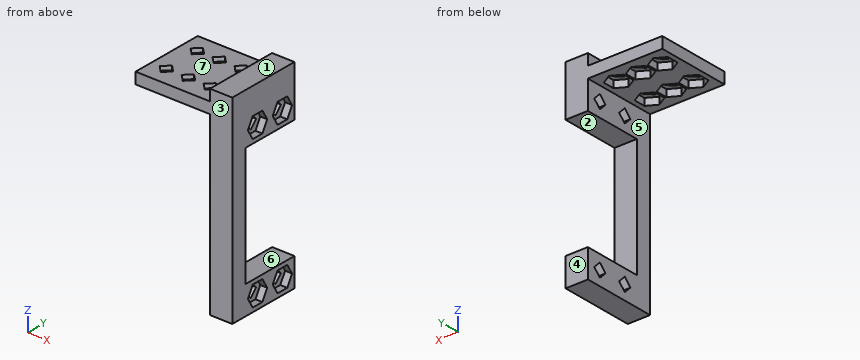
```python
from build123d import *

# Parameters (mm, degrees)
BOSS_EXTRUDE1_DEPTH = 12.7
SKETCH2_W           = 7.62
SKETCH2_H           = 40.64
CUT_EXTRUDE1_DEPTH  = 20
CUT_EXTRUDE2_DEPTH  = 34.02
CUT_EXTRUDE6_DEPTH  = 2.38125
CUT_EXTRUDE5_DEPTH  = 8.62
CUT_EXTRUDE7_DEPTH  = 2.38125
SKETCH14_W          = 25.4
SKETCH14_H          = 3.81
CUT_EXTRUDE8_DEPTH  = 26.4


with BuildPart() as part:
    # Sketch1 → Boss-Extrude1 (new body, symmetric)
    with BuildSketch(Plane(origin=(0, 0, 0), x_dir=(1, 0, 0), z_dir=(0, 1, 0))):
        Polygon((0, 59.944), (0, 0), (-25.4, 0), (-25.4, -7.62), (7.62, -7.62), (7.62, 59.944), align=None)
    extrude(amount=BOSS_EXTRUDE1_DEPTH, both=True)

    # Sketch2 → Cut-Extrude1 (cut)
    with BuildSketch(Plane(origin=(0, 12.7, 0), x_dir=(1, 0, 0), z_dir=(0, 1, 0))):
        with Locations((3.81, 29.972)):
            Rectangle(SKETCH2_W, SKETCH2_H)
    extrude(amount=-CUT_EXTRUDE1_DEPTH, mode=Mode.SUBTRACT)

    # Sketch3 → Cut-Extrude2 (cut, through all)
    with BuildSketch(Plane(origin=(7.62, 0, 0), x_dir=(0, 0, -1), z_dir=(1, 0, 0))):
        Polygon((55.118, 10.087925823), (52.810074177, 7.78), (55.118, 5.472074177), (57.425925823, 7.78), align=None)
        Polygon((2.518074177, 7.78), (4.826, 5.472074177), (7.133925823, 7.78), (4.826, 10.087925823), align=None)
        Polygon((57.425925823, -2.38), (55.118, -0.072074177), (52.810074177, -2.38), (55.118, -4.687925823), align=None)
        Polygon((4.826, -4.687925823), (7.133925823, -2.38), (4.826, -0.072074177), (2.518074177, -2.38), align=None)
    extrude(amount=-CUT_EXTRUDE2_DEPTH, mode=Mode.SUBTRACT)

    # Sketch12 → Cut-Extrude6 (cut)
    with BuildSketch(Plane(origin=(7.62, 0, 0), x_dir=(0, 0, -1), z_dir=(1, 0, 0))):
        Polygon((8.255, 9.759734073), (4.826, 11.739468146), (1.397, 9.759734073), (1.397, 5.800265927), (4.826, 3.820531854), (8.255, 5.800265927), align=None)
        Polygon((4.826, 1.579468146), (1.397, -0.400265927), (1.397, -4.359734073), (4.826, -6.339468146), (8.255, -4.359734073), (8.255, -0.400265927), align=None)
        Polygon((55.118, 1.579468146), (51.689, -0.400265927), (51.689, -4.359734073), (55.118, -6.339468146), (58.547, -4.359734073), (58.547, -0.400265927), align=None)
        Polygon((55.118, 11.739468146), (51.689, 9.759734073), (51.689, 5.800265927), (55.118, 3.820531854), (58.547, 5.800265927), (58.547, 9.759734073), align=None)
    extrude(amount=-CUT_EXTRUDE6_DEPTH, mode=Mode.SUBTRACT)

    # Sketch9 → Cut-Extrude5 (cut, through all)
    with BuildSketch(Plane(origin=(0, 0, 0), x_dir=(-1, 0, 0), z_dir=(0, 0, -1))):
        Polygon((5.196037088, 4.006037088), (7.503962912, 6.313962912), (5.196037088, 8.621888735), (2.888111265, 6.313962912), align=None)
        Polygon((20.203962912, 4.006037088), (22.511888735, 6.313962912), (20.203962912, 8.621888735), (17.896037088, 6.313962912), align=None)
        Polygon((12.7, 4.006037088), (15.007925823, 6.313962912), (12.7, 8.621888735), (10.392074177, 6.313962912), align=None)
    cut_extrude5 = extrude(amount=-CUT_EXTRUDE5_DEPTH, mode=Mode.SUBTRACT)

    # Sketch13 → Cut-Extrude7 (cut)
    with BuildSketch(Plane(origin=(0, 0, 0), x_dir=(-1, 0, 0), z_dir=(0, 0, -1))):
        Polygon((8.625037088, 4.334228839), (8.625037088, 8.293696985), (5.196037088, 10.273431058), (1.767037088, 8.293696985), (1.767037088, 4.334228839), (5.196037088, 2.354494765), align=None)
        Polygon((12.7, 2.354494765), (16.129, 4.334228839), (16.129, 8.293696985), (12.7, 10.273431058), (9.271, 8.293696985), (9.271, 4.334228839), align=None)
        Polygon((20.203962912, 2.354494765), (23.632962912, 4.334228839), (23.632962912, 8.293696985), (20.203962912, 10.273431058), (16.774962912, 8.293696985), (16.774962912, 4.334228839), align=None)
    cut_extrude7 = extrude(amount=-CUT_EXTRUDE7_DEPTH, mode=Mode.SUBTRACT)

    # Mirror2: Cut-Extrude5, Cut-Extrude7 across plane
    add(cut_extrude5.mirror(Plane.ZX), mode=Mode.SUBTRACT)
    add(cut_extrude7.mirror(Plane.ZX), mode=Mode.SUBTRACT)

    # Sketch14 → Cut-Extrude8 (cut, through all)
    with BuildSketch(Plane(origin=(0, 12.7, 0), x_dir=(1, 0, 0), z_dir=(0, 1, 0))):
        with Locations((-12.7, -5.715)):
            Rectangle(SKETCH14_W, SKETCH14_H)
    extrude(amount=-CUT_EXTRUDE8_DEPTH, mode=Mode.SUBTRACT)


solid = part.part
```
CAD build for the part. Positions are in the model's coordinates, mm. Face numbers are marked on the shaded views. A direction names the side the tool comes from. Round coordinates to 2 decimals unless told otherwise and drop trailing zeros. Order: outer loops, then holes, each group sorted by start corner. A loop starts at its lowest first (then second) coordinate and runs counter-clockwise, first axis right, second up. Notation, with made-up numbers: (32, 21) - (61, 21) arc R25 ccw to (61, 38) - close; hole circle Ø3 at (80.5, 71.25). An arc over 180 degrees is marked (long way). Answer as CSV lines item,"result". Start each with the question number.
1. Pull direction Z, two halves, no side cores. Call the marked faces 1, 2 and 3: +Z half, -Z half, draft (parallel to the pull), parting line (faces both ways), or undercut.
2. Tool access for the marked faces 4, 5, 6 and 7: list every direction of +Z, -Z, +X, -X, +Y, -Y with a clear straight run to the whole face (end or side of a thin tool).
3. Saw through at B-B, the plane x = 2. Write the cut outline in (y, z), and give its area (3 significant figures).
4. Saw through at C-C, the plane z = -32.5. Write the cut outline in (x, y).
5. Pin check, flat tips, straight feed: pin 1 (5.5 mm diameter, centred on x = -6.5, y = 7, fed in from -Z); pin 2 (1 mm diameter, centred on x = -10, y = -8, fed in from -Z); pin 3 (6 mm diameter, centred on x = -3.5, y = 5.5, fed in from +Z). Stop position of each tip, or through.
6. Saw through at A-A, the plane z = -6. Write the cut outline in (x, y).
7. Drill centre lines: L1, parallel to X at y = 2.75, z = 1; L2, parallel to X at y = -9.75, z = -2; L3, parallel to Z at x = -15.5, y = -10.25. Where is each one in solid material? Low to high. Write a range as [from, to].
Model answer:
1,face 1,"+Z half"
1,face 2,"undercut"
1,face 3,"draft"
2,face 4,"+Z, -Z, +X, -X, +Y"
2,face 5,"-Z, -X, +Y, -Y"
2,face 6,"+X, -X, +Y"
2,face 7,"+Z, -X, +Y, -Y"
3,outline,"(-12.7, -59.94) - (12.7, -59.94) - (12.7, -50.29) - (-7.3, -50.29) - (-7.3, -9.65) - (12.7, -9.65) - (12.7, 7.62) - (-12.7, 7.62) - close; hole (-4.69, -55.12) - (-2.38, -57.43) - (-0.07, -55.12) - (-2.38, -52.81) - close; hole (-4.69, -4.83) - (-2.38, -7.13) - (-0.07, -4.83) - (-2.38, -2.52) - close; hole (5.47, -55.12) - (7.78, -57.43) - (10.09, -55.12) - (7.78, -52.81) - close; hole (5.47, -4.83) - (7.78, -7.13) - (10.09, -4.83) - (7.78, -2.52) - close"
3,area,"861 mm²"
4,outline,"(0, -12.7) - (7.62, -12.7) - (7.62, -7.3) - (0, -7.3) - close"
5,pin 1,"stops at z = 0"
5,pin 2,"stops at z = 2.38"
5,pin 3,"stops at z = 3.81"
6,outline,"(0, -12.7) - (7.62, -12.7) - (7.62, -5.66) - (5.24, -5.66) - (5.24, -3.51) - (0, -3.51) - close; (0, -1.25) - (5.24, -1.25) - (5.24, 0.9) - (7.62, 0.9) - (7.62, 4.5) - (5.24, 4.5) - (5.24, 6.65) - (0, 6.65) - close; (0, 8.91) - (5.24, 8.91) - (5.24, 11.06) - (7.62, 11.06) - (7.62, 12.7) - (0, 12.7) - close"
7,L1,"x = [-25.4, -20.89], [-19.52, -13.39], [-12.01, -5.88], [-4.51, 7.62]"
7,L2,"x = [0, 7.62]"
7,L3,"z = [0, 3.81]"
